from build123d import *

# Parameters (mm, degrees)
SKETCH1_R           = 66
SKETCH1_R_2         = 54
SKETCH1_R_3         = 4.25
BOSS_EXTRUDE1_DEPTH = 5


with BuildPart() as part:
    # Sketch1 → Boss-Extrude1 (new body)
    with BuildSketch(Plane(origin=(0, 0, 0), x_dir=(1, 0, 0), z_dir=(0, 1, 0))):
        Circle(SKETCH1_R)
        Circle(SKETCH1_R_2, mode=Mode.SUBTRACT)
        with Locations((0, 60)):
            Circle(SKETCH1_R_3, mode=Mode.SUBTRACT)
        with Locations((11.705419321, 58.847116824)):
            Circle(SKETCH1_R_3, mode=Mode.SUBTRACT)
        with Locations((22.961005942, 55.432771951)):
            Circle(SKETCH1_R_3, mode=Mode.SUBTRACT)
        with Locations((33.334213981, 49.888176738)):
            Circle(SKETCH1_R_3, mode=Mode.SUBTRACT)
        with Locations((42.426406871, 42.426406871)):
            Circle(SKETCH1_R_3, mode=Mode.SUBTRACT)
        with Locations((49.888176738, 33.334213981)):
            Circle(SKETCH1_R_3, mode=Mode.SUBTRACT)
        with Locations((55.432771951, 22.961005942)):
            Circle(SKETCH1_R_3, mode=Mode.SUBTRACT)
        with Locations((58.847116824, 11.705419321)):
            Circle(SKETCH1_R_3, mode=Mode.SUBTRACT)
        with Locations((60, 0)):
            Circle(SKETCH1_R_3, mode=Mode.SUBTRACT)
        with Locations((58.847116824, -11.705419321)):
            Circle(SKETCH1_R_3, mode=Mode.SUBTRACT)
        with Locations((55.432771951, -22.961005942)):
            Circle(SKETCH1_R_3, mode=Mode.SUBTRACT)
        with Locations((49.888176738, -33.334213981)):
            Circle(SKETCH1_R_3, mode=Mode.SUBTRACT)
        with Locations((42.426406871, -42.426406871)):
            Circle(SKETCH1_R_3, mode=Mode.SUBTRACT)
        with Locations((33.334213981, -49.888176738)):
            Circle(SKETCH1_R_3, mode=Mode.SUBTRACT)
        with Locations((22.961005942, -55.432771951)):
            Circle(SKETCH1_R_3, mode=Mode.SUBTRACT)
        with Locations((11.705419321, -58.847116824)):
            Circle(SKETCH1_R_3, mode=Mode.SUBTRACT)
        with Locations((0, -60)):
            Circle(SKETCH1_R_3, mode=Mode.SUBTRACT)
        with Locations((-11.705419321, -58.847116824)):
            Circle(SKETCH1_R_3, mode=Mode.SUBTRACT)
        with Locations((-22.961005942, -55.432771951)):
            Circle(SKETCH1_R_3, mode=Mode.SUBTRACT)
        with Locations((-33.334213981, -49.888176738)):
            Circle(SKETCH1_R_3, mode=Mode.SUBTRACT)
        with Locations((-42.426406871, -42.426406871)):
            Circle(SKETCH1_R_3, mode=Mode.SUBTRACT)
        with Locations((-49.888176738, -33.334213981)):
            Circle(SKETCH1_R_3, mode=Mode.SUBTRACT)
        with Locations((-55.432771951, -22.961005942)):
            Circle(SKETCH1_R_3, mode=Mode.SUBTRACT)
        with Locations((-58.847116824, -11.705419321)):
            Circle(SKETCH1_R_3, mode=Mode.SUBTRACT)
        with Locations((-60, 0)):
            Circle(SKETCH1_R_3, mode=Mode.SUBTRACT)
        with Locations((-58.847116824, 11.705419321)):
            Circle(SKETCH1_R_3, mode=Mode.SUBTRACT)
        with Locations((-55.432771951, 22.961005942)):
            Circle(SKETCH1_R_3, mode=Mode.SUBTRACT)
        with Locations((-49.888176738, 33.334213981)):
            Circle(SKETCH1_R_3, mode=Mode.SUBTRACT)
        with Locations((-42.426406871, 42.426406871)):
            Circle(SKETCH1_R_3, mode=Mode.SUBTRACT)
        with Locations((-33.334213981, 49.888176738)):
            Circle(SKETCH1_R_3, mode=Mode.SUBTRACT)
        with Locations((-22.961005942, 55.432771951)):
            Circle(SKETCH1_R_3, mode=Mode.SUBTRACT)
        with Locations((-11.705419321, 58.847116824)):
            Circle(SKETCH1_R_3, mode=Mode.SUBTRACT)
    extrude(amount=BOSS_EXTRUDE1_DEPTH)


solid = part.part
Geometry check sheet. Reference: the model listing, model coordinates, mm. Give positions to 0.01 mm unless a question says otherwise; leave off trailing zeros. Loops run counter-clockwise (first coordinate to the right, second up) from the corner with the lowest first, then second, coordinate; pieces in that order, holes last. Notation, with made-up numbers: M 79,61 L 131,61 A13 cw 131,75 Z; hole C 34,43 d8. An arc over 180 degrees is marked long. Answer as a JSON object with one key per item and string values. Group by question number.
Item 1: Mould release check, pull along X, two halves, no side actions. Record for faces 1 (the cylindrical face through (60.967, 2.465, 25.278)), 2 (the cylindrical face through (46.48, 2.46, 41.15)), 3 (the flat face through (-54, 5, 5)): pulls with the +X half, pulls with the -X half, needs draft (parallel to the pull), parting line crosses it, or undercut.
Item 2: Sectioned sample at A-A on x = 0. Record the boundary of the cut face in (y, z), plus the area to 3 significant figures.
Item 3: Sectioned sample at C-C on y = 1.65. Give the number of separate pieces and of enclosed holes in the cut face, plus the area to 3 significant figures.
Item 4: Sectioned sample at B-B on z = 0. Record the boundary of the cut face in (x, y), plus the area to 3 significant figures.
Item 5: Gauge pin test, flat ends, axial feed: pin 1 (11 mm diameter, centred on x = -49.89, z = -33.33, fed in from -Y); pin 2 (3 mm diameter, centred on y = 3.5, z = -16.5, fed in from +X); pin 3 (1 mm diameter, centred on y = 4.5, z = -46.5, fed in from +X); pin 4 (3 mm diameter, centred on y = 1, z = 41.5, fed in from -X). Record the tip position at first contact, or that the pin passes through.
Item 6: Material ranges on L1, parallel to X at y = 1.7, z = 0; L2, parallel to X at y = 1, z = -20; L3, parallel to Z at x = -36, y = 2.25, recorded low to high.
Findings below:
{
 "1": {"face 1": "parting line crosses it", "face 2": "undercut", "face 3": "needs draft"},
 "2": {"outline": "M 0,-66 L 5,-66 L 5,-64.25 L 0,-64.25 Z; M 0,-55.75 L 5,-55.75 L 5,-54 L 0,-54 Z; M 0,54 L 5,54 L 5,55.75 L 0,55.75 Z; M 0,64.25 L 5,64.25 L 5,66 L 0,66 Z", "area": "35.0 mm2"},
 "3": {"separate pieces": "1", "enclosed holes": "33", "area": "2,710 mm2"},
 "4": {"outline": "M -66,0 L -64.25,0 L -64.25,5 L -66,5 Z; M -55.75,0 L -54,0 L -54,5 L -55.75,5 Z; M 54,0 L 55.75,0 L 55.75,5 L 54,5 Z; M 64.25,0 L 66,0 L 66,5 L 64.25,5 Z", "area": "35.0 mm2"},
 "5": {"pin 1": "y = 0", "pin 2": "x = 64.27", "pin 3": "x = 47.33", "pin 4": "x = -52.5"},
 "6": {"L1": "-66 to -64.25, -55.75 to -54, 54 to 55.75, 64.25 to 66", "L2": "-62.9 to -58.48, -52.38 to -50.16, 50.16 to 52.38, 58.48 to 62.9", "L3": "-55.32 to -53.2, -46.58 to -40.25, 40.25 to 46.58, 53.2 to 55.32"}
}
